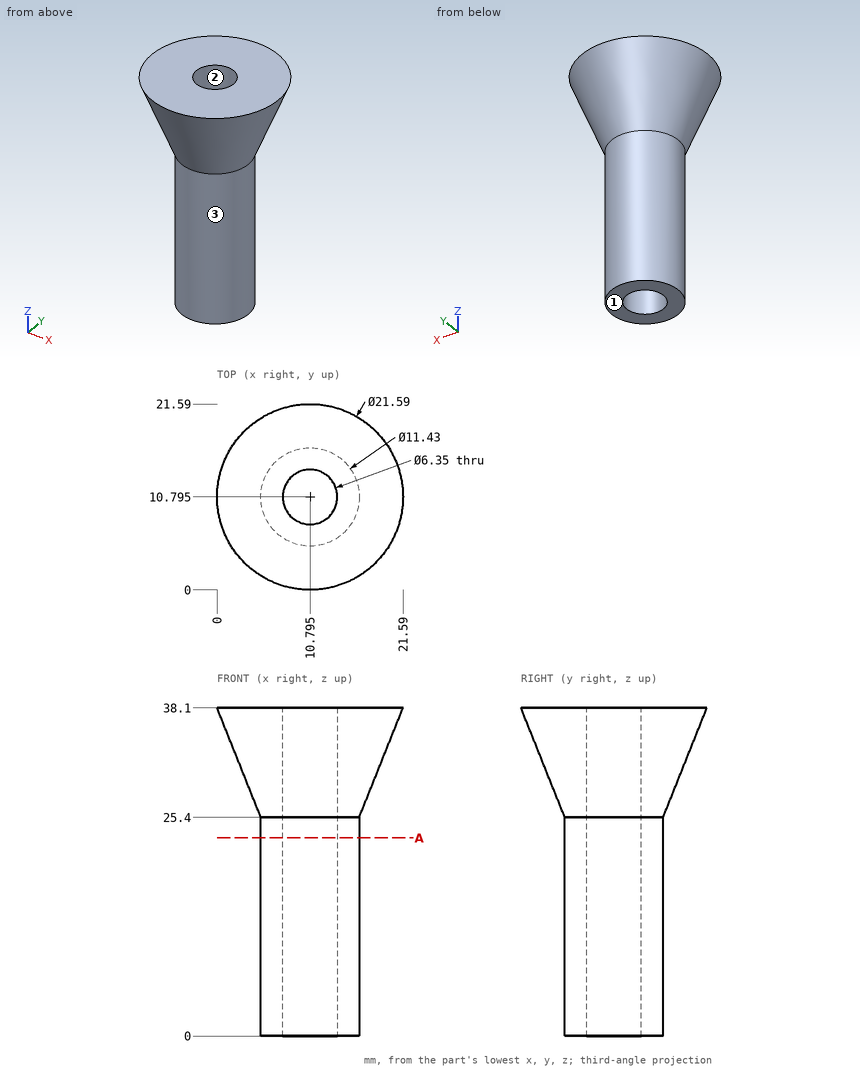
For this review, use the dimensioned drawing (mm, ordinates from the lowest corner) and the shaded views. Give positions to 0.01 mm unless a question says otherwise; leave off trailing zeros. Order: outer loops, then holes, each group sorted by start corner. A loop starts at its lowest first (then second) coordinate and runs counter-clockwise, first axis right, second up.
1) Insertion check: pin 1 (1 mm diameter, centred on x = 17, z = 28.5, fed in from -Y); pin 2 (2 mm diameter, centred on y = 13.5, z = 10, fed in from +X); pin 3 (8 mm diameter, centred on x = 9, y = 8.5, fed in from -Z); pin 4 (4 mm diameter, centred on x = 10.795, y = 10.795, fed in from +Z). Each pin has a flat end and moves straight along its axis. Give the tip position at first contact, or say it passes through.
2) Take a section at A-A (z = 23). Give the boundary of the cut face in (x, y) (3 decimals), then the cut area to 3 significant figures.
3) The part is to be moulded in two halves that separate along X. For the marked faces 1, 2 and 3, say which applies: released by +X, released by -X, zero draft, split by the parting line, or undercut.
4) Wall thickness on line 1 (Y direction, x = 11, z = 21); line 2 (X direction, y = 11.75, z = 25); line 3 (X direction, y = 11.5, z = 13): over which ranges is each line inside the solid? List them lowest first.
Derived:
1. pin 1: stops at y = 6.74
1. pin 2: stops at x = 16.25
1. pin 3: stops at z = 0
1. pin 4: passes through
2. outline: circle Ø11.43 at (10.795, 10.795); hole circle Ø6.35 at (10.795, 10.795)
2. area: 70.9 mm2
3. face 1: zero draft
3. face 2: undercut
3. face 3: split by the parting line
4. line 1: y = 5.08 to 7.63, 13.96 to 16.51
4. line 2: x = 5.16 to 7.77, 13.82 to 16.43
4. line 3: x = 5.12 to 7.7, 13.89 to 16.47
